Geometry: see drawing. Coordinates: mm, zero at the bounding-box minimum. Coordinates: 2 decimals unless noted, no trailing zeros. Order: outer loops, then holes, each group sorted by start corner. A loop starts at its lowest first (then second) coordinate and runs counter-clockwise, first axis right, second up.
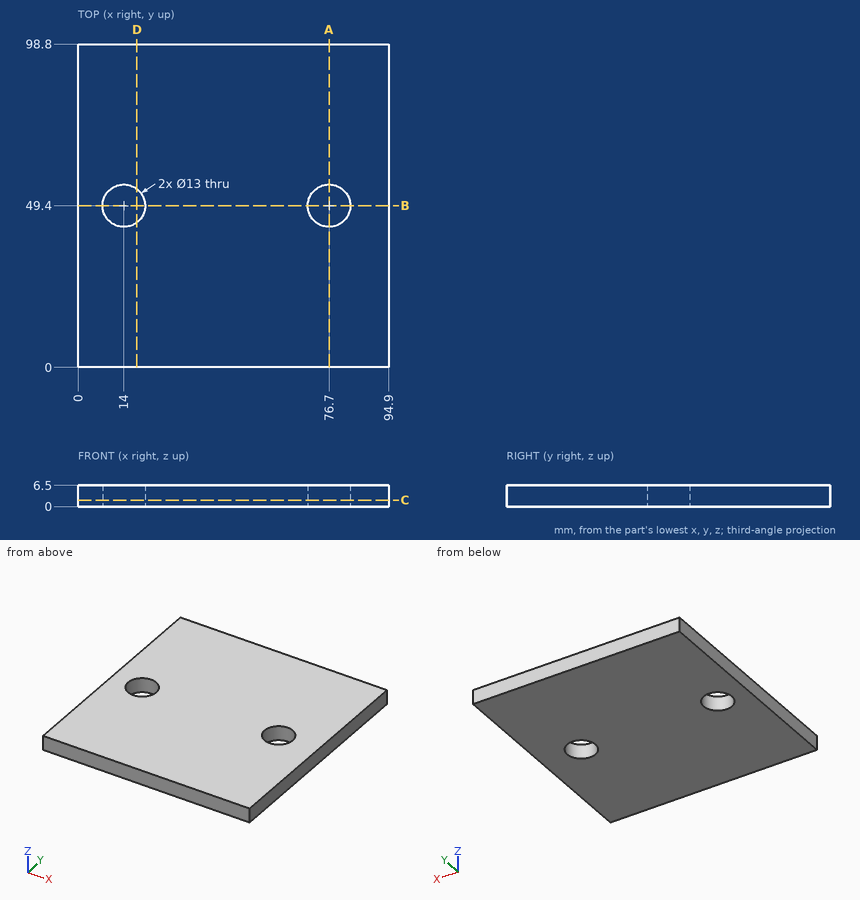
Item 1: Ray query, probe 1 along X at (y, z) = (49.4, 5); probe 2 along Y at (x, z) = (13.5, 5.5); probe 3 along X at (y, z) = (54.5, 1.5). Return the intervals inside material, ascending.
Response values:
probe 1: x = 0 to 7.5, 20.5 to 70.2, 83.2 to 94.9
probe 2: y = 0 to 42.92, 55.88 to 98.8
probe 3: x = 0 to 9.97, 18.03 to 72.67, 80.73 to 94.9
Item 2: Cut plane C-C on z = 2. Return loops of the section in (x, y).
Response values:
outline: (0, 0) - (94.9, 0) - (94.9, 98.8) - (0, 98.8) - close; hole circle Ø13 at (14, 49.4); hole circle Ø13 at (76.7, 49.4)
Item 3: Cut plane D-D on x = 18. Return loops of the section in (y, z), then the cut area to 3 significant figures.
Response values:
outline: (0, 0) - (44.28, 0) - (44.28, 6.5) - (0, 6.5) - close; (54.52, 0) - (98.8, 0) - (98.8, 6.5) - (54.52, 6.5) - close
area: 576 mm2
Item 4: Cut plane A-A on x = 76.7. Return loops of the section in (y, z), then the cut area to 3 significant figures.
Response values:
outline: (0, 0) - (42.9, 0) - (42.9, 6.5) - (0, 6.5) - close; (55.9, 0) - (98.8, 0) - (98.8, 6.5) - (55.9, 6.5) - close
area: 558 mm2
Item 5: Cut plane B-B on y = 49.4. Return loops of the section in (x, z).
Response values:
outline: (0, 0) - (7.5, 0) - (7.5, 6.5) - (0, 6.5) - close; (20.5, 0) - (70.2, 0) - (70.2, 6.5) - (20.5, 6.5) - close; (83.2, 0) - (94.9, 0) - (94.9, 6.5) - (83.2, 6.5) - close
